Verification items for the finished model (mm, model axes). Face numbers are marked on the shaded views. A direction names the side the tool comes from. Coordinates: 2 decimals unless noted, no trailing zeros. Order: outer loops, then holes, each group sorted by start corner. A loop starts at its lowest first (then second) coordinate and runs counter-clockwise, first axis right, second up. Notation, with made-up numbers: M -35.75,6.25 L -26.75,6.25 A27 ccw -26.75,23.25 Z; hole C 47,-8.75 d2. An arc over 180 degrees is marked long. Use one line per item in the form item = value. Start each with the question number.
```python
from build123d import *

# Parameters (mm, degrees)
F1_DEPTH = 25
F2_R     = 2.25
F3_DEPTH = 25
F4_R     = 3.5
F4_R_2   = 2.12
F5_DEPTH = 25


with BuildPart() as f1:
    # F0 (on Top) → F1 (new body)
    with BuildSketch(Plane.XY):
        with BuildLine():
            ThreePointArc((-2, -31), (-0.585786, -30.414214), (0, -29))
            Line((0, -29), (0, -4))
            ThreePointArc((0, -4), (1.171573, -1.171573), (4, 0))
            Line((4, 0), (57, 0))
            ThreePointArc((57, 0), (57.707107, 0.292893), (58, 1))
            Line((58, 1), (58, 2))
            ThreePointArc((58, 2), (57.707107, 2.707107), (57, 3))
            Line((57, 3), (-3, 3))
            Line((-3, 3), (-3, -31))
            Line((-3, -31), (-2, -31))
        make_face()
    extrude(amount=F1_DEPTH)

    # F2 (on face) → F3 (cut)
    with BuildSketch(Plane.YZ):
        with Locations((-22.75, 18.75)):
            Circle(F2_R)
        with Locations((-10.25, 18.75)):
            Circle(F2_R)
        with Locations((-10.25, 6.25)):
            Circle(F2_R)
        with Locations((-22.75, 6.25)):
            Circle(F2_R)
    extrude(amount=-F3_DEPTH, mode=Mode.SUBTRACT)

    # F4 (on face) → F5 (cut)
    with BuildSketch(Plane.XZ):
        with Locations((42.66, 8.5)):
            Circle(F4_R)
        with Locations((50.88, 16.71316)):
            Circle(F4_R_2)
        with Locations((34.44, 16.71316)):
            Circle(F4_R_2)
    extrude(amount=-F5_DEPTH, mode=Mode.SUBTRACT)


solid = f1.part
```
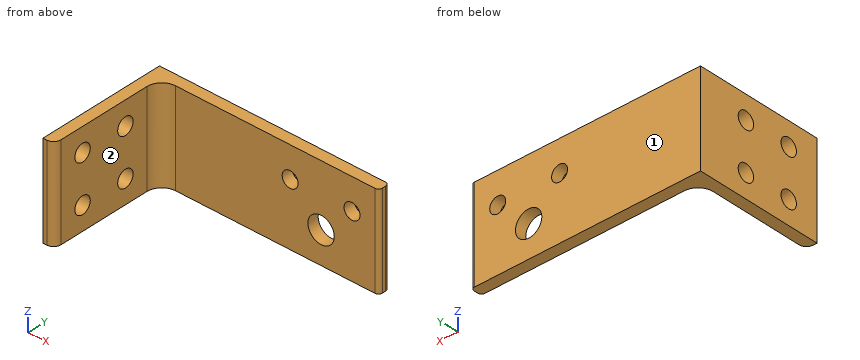
1. Cross-section at A-A on y = -22.75. Enter the section's corners in (x, z), and give its area (3 significant figures).
2. Material ranges on line 1 along Y through (x, z) = (12, 14); line 2 along X through (y, z) = (-20, 13.75); line 3 along Z through (x, y) = (42.66, 1), recorded low to high.
3. Tool access check on the marked faces 1 and 2. Record the directions out of +Z, -Z, +X, -X, +Y, -Y that give a thin tool (end or side, any length) a straight path to the whole face; none if there is none.
4. Cross-section at C-C on z = 17.5. Enter the section's corners in (x, y).
5. Cross-section at B-B on x = 34.44. Enter the section's corners in (y, z).
6. Depth check by flat-ended pin: P1, Ø6, axis at y = -22.75, z = 6.25, coming from the +X side; P2, Ø1.5, axis at x = 21, z = 19, coming from the -Y side; P3, Ø5, axis at x = 50.88, z = 16.71, coming from the +Y side. Enter the tip coordinate at first touch or a pass-through.
7. Cross-section at D-D on z = 6.25. Enter the section's corners in (x, y).
Final values:
q1.outline = M -3,0 L 0,0 L 0,4 L -3,4 Z; M -3,8.5 L 0,8.5 L 0,16.5 L -3,16.5 Z; M -3,21 L 0,21 L 0,25 L -3,25 Z
q1.area = 48.0 mm2
q2.line_1 = 0 to 3
q2.line_2 = -3 to 0
q2.line_3 = 0 to 5, 12 to 25
q3.face_1 = +Z, -Z, +X, -X, +Y
q3.face_2 = +Z, -Z, +X, -Y
q4.outline = M -3,-31 L -2,-31 A2 ccw 0,-29 L 0,-24.62 L -3,-24.62 Z; M -3,-20.88 L 0,-20.88 L 0,-12.12 L -3,-12.12 Z; M -3,-8.38 L 0,-8.38 L 0,-4 A4 cw 4,0 L 32.47,0 L 32.47,3 L -3,3 Z; M 36.41,0 L 48.91,0 L 48.91,3 L 36.41,3 Z; M 52.85,0 L 57,0 A1 ccw 58,1 L 58,2 A1 ccw 57,3 L 52.85,3 Z
q5.outline = M 0,0 L 3,0 L 3,14.59 L 0,14.59 Z; M 0,18.83 L 3,18.83 L 3,25 L 0,25 Z
q6.P1 = 0
q6.P2 = 0
q6.P3 = 3
q7.outline = M -3,-31 L -2,-31 A2 ccw 0,-29 L 0,-25 L -3,-25 Z; M -3,-20.5 L 0,-20.5 L 0,-12.5 L -3,-12.5 Z; M -3,-8 L 0,-8 L 0,-4 A4 cw 4,0 L 39.98,0 L 39.98,3 L -3,3 Z; M 45.34,0 L 57,0 A1 ccw 58,1 L 58,2 A1 ccw 57,3 L 45.34,3 Z
